from build123d import *

# Parameters (mm, degrees)
CHANFREIN1_SIZE = 0.5
CHANFREIN2_SIZE = 1
CHANFREIN3_SIZE = 0.2


with BuildPart() as part:
    # Esquisse1 → Base-Révolution (revolve)
    with BuildSketch(Plane.XY, mode=Mode.PRIVATE) as base_r_volution_sk:
        Polygon((12.5, 10.5), (16.5, 10.5), (16.5, 5.5), (0, 5.5), (0, 8), (12.5, 8), align=None)
    revolve(base_r_volution_sk.sketch.rotate(Axis((11.390827922, 0, 0), (1, 0, 0)), 90), axis=Axis((11.390827922, 0, 0), (1, 0, 0)))

    # Chanfrein1
    chanfrein1_edges = [part.edges().sort_by_distance(p)[0] for p in [
        (16.5, 0, -10.5),
    ]]
    chamfer(chanfrein1_edges, length=CHANFREIN1_SIZE)

    # Chanfrein2
    chanfrein2_edges = [part.edges().sort_by_distance(p)[0] for p in [
        (0, 0, -8),
    ]]
    chamfer(chanfrein2_edges, length=CHANFREIN2_SIZE)

    # Chanfrein3
    chanfrein3_edges = [part.edges().sort_by_distance(p)[0] for p in [
        (0, 0, -5.5),
        (16.5, 0, -5.5),
    ]]
    chamfer(chanfrein3_edges, length=CHANFREIN3_SIZE)


solid = part.part
For this review, take the finished solid that the model builds, in its own axes (mm). A direction names the side the tool comes from. Round coordinates to 2 decimals unless told otherwise and drop trailing zeros. Order: outer loops, then holes, each group sorted by start corner. A loop starts at its lowest first (then second) coordinate and runs counter-clockwise, first axis right, second up. Notation, with made-up numbers: M 65,28 L 95,28 A25 cw 95,49 Z; hole C -38.75,-12.75 d7. An arc over 180 degrees is marked long. Use a Markdown table: item, result. Add a question column.
Item 1: Tool access review of faces 1 (the cylindrical face through (6.83, 7.81, -1.73)), 2 (the flat face through (16.5, 4.3, 4.3)): name each direction out of +Z, -Z, +X, -X, +Y, -Y from which nothing blocks a thin tool from reaching the whole face with its end or side.
Item 2: Add section D-D, the plane x = 13.75. Give the boundary of the cut face in (y, z), then the cut area to 3 significant figures.
Item 3: Add section A-A, the plane y = 0. Give the boundary of the cut face in (x, z), then the cut area to 3 significant figures.
Item 4: To check wall thickness, follow line 1 along Y through (x, z) = (9.25, 0); line 2 along Y through (x, z) = (9.5, -4.25); line 3 along X through (y, z) = (-4.5, 8.5). State the ranges of each line that lie inside material, in increasing order.
Item 5: Insertion check: pin 1 (6 mm diameter, centred on x = 3.5, z = -1.5, fed in from -Y); pin 2 (2 mm diameter, centred on x = 12, y = -3.5, fed in from -Z); pin 3 (2 mm diameter, centred on y = -3.5, z = 2.5, fed in from -X); pin 4 (1 mm diameter, centred on x = 3, z = -3, fed in from -Y). Each pin has a flat end and moves straight along its axis. Give the tip position at first contact, or say it passes through.
Item 6: Mouldability with a two-part tool opening along Z and no side actions: class faces 3 (the cylindrical face through (8.14, 5.37, -1.19)), 4 (the cylindrical face through (14.3, -3.2, 10)), 5 (the flat face through (0, 0, 6)) as released by +Z, released by -Z, zero draft, split by the parting line, or undercut.
Item 7: Add section C-C, the plane x = 4.75. Give the boundary of the cut face in (y, z), then the cut area to 3 significant figures.
Geometry results:
| question | item | result |
|---|---|---|
| 1 | face 1 | -X |
| 1 | face 2 | +Z, -Z, +X, +Y, -Y |
| 2 | outline | C 0,0 d21; hole C 0,0 d11 |
| 2 | area | 251 mm² |
| 3 | outline | M 0,-7 L 1,-8 L 12.5,-8 L 12.5,-10.5 L 16,-10.5 L 16.5,-10 L 16.5,-5.7 L 16.3,-5.5 L 0.2,-5.5 L 0,-5.7 Z; M 0,5.7 L 0.2,5.5 L 16.3,5.5 L 16.5,5.7 L 16.5,10 L 16,10.5 L 12.5,10.5 L 12.5,8 L 1,8 L 0,7 Z |
| 3 | area | 101 mm² |
| 4 | line 1 | y = -8 to -5.5, 5.5 to 8 |
| 4 | line 2 | y = -6.78 to -3.49, 3.49 to 6.78 |
| 4 | line 3 | x = 12.5 to 16.5 |
| 5 | pin 1 | stops at y = -8 |
| 5 | pin 2 | stops at z = -10.16 |
| 5 | pin 3 | passes through |
| 5 | pin 4 | stops at y = -7.6 |
| 6 | face 3 | undercut |
| 6 | face 4 | split by the parting line |
| 6 | face 5 | zero draft |
| 7 | outline | C 0,0 d16; hole C 0,0 d11 |
| 7 | area | 106 mm² |
